Input: part model. Units: mm. Frame: model coordinates. A direction names the side the tool comes from. Round coordinates to 2 decimals unless told otherwise and drop trailing zeros. Order: outer loops, then holes, each group sorted by start corner. A loop starts at its lowest first (then second) coordinate and runs counter-clockwise, first axis right, second up. Notation, with made-up numbers: (53.5, 71) -> (68.5, 71) arc R21 cw to (68.5, 86) -> close; hole circle Ø7 at (-20, 23). An arc over 180 degrees is marked (long way). Use a Markdown table: item, result.
from build123d import *

# Parameters (mm, degrees)
SKETCH5_W             = 49.6
SKETCH5_H             = 24.3
SKETCH5_W_2           = 43.6
SKETCH5_H_2           = 18.3
BOSS_EXTRUDE3_DEPTH   = 7.5
FILLET1_R             = 3
SKETCH7_W             = 2.5
SKETCH7_H             = 2.5
BOSS_EXTRUDE5_DEPTH   = 4
SKETCH11_W            = 10
SKETCH11_H            = 4
BOSS_EXTRUDE6_DEPTH   = 12
FILLET3_R             = 3
SKETCH13_R            = 2.25
CUT_EXTRUDE1_DEPTH    = 56.377341937
CHAMFER2_SIZE         = 1
CHAMFER2_SIZE2        = 1.732050808
CIRPATTERN1_OUTLINE_R = 2.25
CIRPATTERN1_DEPTH     = 2.9999999
CIRPATTERN1_START     = 2.9999999
CIRPATTERN1_2_DEPTH   = 1.0000001
FILLET5_R             = 3
FILLET6_R             = 1


with BuildPart() as part:
    # Sketch5 → Boss-Extrude3 (new body)
    with BuildSketch(Plane(origin=(0, 0, 0), x_dir=(1, 0, 0), z_dir=(0, 1, 0))):
        with Locations((24.8, 12.15)):
            Rectangle(SKETCH5_W, SKETCH5_H)
        with Locations((24.8, 12.15)):
            Rectangle(SKETCH5_W_2, SKETCH5_H_2, mode=Mode.SUBTRACT)
    extrude(amount=BOSS_EXTRUDE3_DEPTH)

    # Fillet1
    fillet1_edges = [part.edges().sort_by_distance(p)[0] for p in [
        (49.6, 3.75, -24.3),
        (49.6, 3.75, 0),
        (0, 3.75, 0),
        (0, 3.75, -24.3),
    ]]
    fillet(fillet1_edges, radius=FILLET1_R)

    # Sketch7 → Boss-Extrude5 (add)
    with BuildSketch(Plane(origin=(0, 0, 0), x_dir=(1, 0, 0), z_dir=(0, 1, 0))):
        with Locations((45.35, 4.25)):
            Rectangle(SKETCH7_W, SKETCH7_H)
        with Locations((45.35, 20.05)):
            Rectangle(SKETCH7_W, SKETCH7_H)
        with Locations((4.25, 4.25)):
            Rectangle(SKETCH7_W, SKETCH7_H)
        with Locations((4.25, 20.05)):
            Rectangle(SKETCH7_W, SKETCH7_H)
    extrude(amount=BOSS_EXTRUDE5_DEPTH)

    # Sketch11 → Boss-Extrude6 (add)
    with BuildSketch(Plane.XY):
        with Locations((24.8, 2)):
            Rectangle(SKETCH11_W, SKETCH11_H)
    extrude(amount=BOSS_EXTRUDE6_DEPTH)

    # Fillet3
    fillet3_edges = [part.edges().sort_by_distance(p)[0] for p in [
        (19.8, 2, 0),
        (29.8, 2, 0),
        (24.8, 4, 0),
        (19.8, 2, 12),
        (29.8, 2, 12),
    ]]
    fillet(fillet3_edges, radius=FILLET3_R)

    # Sketch13 → Cut-Extrude1 (cut, through all)
    with BuildSketch(Plane(origin=(0, 4, 0), x_dir=(1, 0, 0), z_dir=(0, 1, 0))):
        with Locations(Location((24.8, -7, 0), (0, 0, 270))):
            Circle(SKETCH13_R)
    extrude(amount=-CUT_EXTRUDE1_DEPTH, mode=Mode.SUBTRACT)

    # Chamfer2
    chamfer2_edges = [part.edges().sort_by_distance(p)[0] for p in [
        (24.8, 4, 4.75),
    ]]
    chamfer2_side = [part.faces().sort_by_distance(p)[0] for p in [
        (24.8, 2, 4.75),
    ]]
    chamfer(chamfer2_edges, length=CHAMFER2_SIZE, length2=CHAMFER2_SIZE2, reference=chamfer2_side[0])

    # CirPattern1: read off the stored shape, not the designer's step
    # CirPattern1 outline → CirPattern1 (add)
    with BuildSketch(Plane(origin=(0, 0, 0), x_dir=(1, 0, 0), z_dir=(0, 1, 0))):
        with BuildLine():
            Line((19.8, 33.3), (19.8, 24.3))
            Line((19.8, 24.3), (29.8, 24.3))
            Line((29.8, 24.3), (29.8, 33.3))
            ThreePointArc((29.8, 33.3), (28.921320344, 35.421320344), (26.8, 36.3))
            Line((26.8, 36.3), (22.8, 36.3))
            ThreePointArc((22.8, 36.3), (20.678679656, 35.421320344), (19.8, 33.3))
        make_face()
        with Locations((24.8, 31.3)):
            Circle(CIRPATTERN1_OUTLINE_R, mode=Mode.SUBTRACT)
    extrude(amount=CIRPATTERN1_DEPTH)

    # CirPattern1 2 outline → CirPattern1 2 (add)
    with BuildSketch(Plane(origin=(0, 0, 0), x_dir=(1, 0, 0), z_dir=(0, 1, 0)).offset(CIRPATTERN1_START)):
        with BuildLine():
            Line((19.8, 33.3), (19.8, 24.3))
            Line((19.8, 24.3), (29.8, 24.3))
            Line((29.8, 24.3), (29.8, 33.3))
            ThreePointArc((29.8, 33.3), (28.921320344, 35.421320344), (26.8, 36.3))
            Line((26.8, 36.3), (22.8, 36.3))
            ThreePointArc((22.8, 36.3), (20.678679656, 35.421320344), (19.8, 33.3))
        make_face()
    extrude(amount=CIRPATTERN1_2_DEPTH)

    # CirPattern1 3 outline → CirPattern1 3 (revolve, cut)
    with BuildSketch(Plane(origin=(24.8, 0, -31.3), x_dir=(1, 0, 0), z_dir=(0, 0, 1))):
        Polygon((0, 2.9999999), (2.25, 2.9999999), (3.982050808, 4), (0, 4), align=None)
    revolve(axis=Axis((24.8, 0, -31.3), (0, 1, 0)), mode=Mode.SUBTRACT)

    # Fillet5
    fillet5_edges = [part.edges().sort_by_distance(p)[0] for p in [
        (29.8, 2, -24.3),
        (19.8, 2, -24.3),
        (24.8, 4, -24.3),
    ]]
    fillet(fillet5_edges, radius=FILLET5_R)

    # Fillet6
    fillet6_edges = [part.edges().sort_by_distance(p)[0] for p in [
        (5.5, 2, -18.8),
        (5.5, 2, -5.5),
        (44.1, 2, -5.5),
        (44.1, 2, -18.8),
    ]]
    fillet(fillet6_edges, radius=FILLET6_R)


solid = part.part
1) Pull-direction query (X, two-part tool) for faces 1 (the flat face through (46.6, 4, -12)), 2 (the cylindrical face through (31.11, 2.77, -24.82)), 3 (the flat face through (44.1, 2, -21)), 4 (the cylindrical face through (18.49, 2.77, 0.52)); classes: +X half, -X half, draft (parallel to the pull), parting line (faces both ways), or undercut.
Results found:
| item | result |
|---|---|
| face 1 | undercut |
| face 2 | +X half |
| face 3 | undercut |
| face 4 | -X half |
2) Cut plane B-B on z = 7. Return loops of the section in (x, y).
Results found:
| item | result |
|---|---|
| outline | (19.8, 0) -> (22.55, 0) -> (22.55, 3) -> (20.82, 4) -> (19.8, 4) -> close; (27.05, 0) -> (29.8, 0) -> (29.8, 4) -> (28.78, 4) -> (27.05, 3) -> close |
3) Set-up query: faces 5 (the flat face through (45, 4, -20)), 6 (the flat face through (19.8, 2, -30)), 7 (the flat face through (4, 2, -5.5)), 8 (the flat face through (19.8, 2, 6)). Return all of +Z, -Z, +X, -X, +Y, -Y with unobstructed straight access to the full face (end or side cutting, diameter ignored); none if empty.
Results found:
| item | result |
|---|---|
| face 5 | +Y |
| face 6 | -Z, -X, +Y, -Y |
| face 7 | +Y, -Y |
| face 8 | +Z, -X, +Y, -Y |
4) Pin query (flat end, axial travel): pin 1 Ø3 at (x, y) = (37, 6) entering from -Z; pin 2 Ø3 at (y, z) = (2, 5.5) entering from -X; pin 3 Ø2.5 at (x, z) = (24.8, 7) entering from +Y; pin 4 Ø4.5 at (x, z) = (27, -32.5) entering from +Y. Return the tip coordinate at first contact, or that it passes through.
Results found:
| item | result |
|---|---|
| pin 1 | stops at z = -24.3 |
| pin 2 | stops at x = 19.8 |
| pin 3 | passes through |
| pin 4 | stops at y = 4 |
5) Line query: L1, parallel to Z at x = 11.5, y = 3; L2, parallel to X at y = 0.75, z = 7; L3, parallel to Z at x = 32, y = 4. Output: solid intervals per line, ascending. Write a range as [from, to].
Results found:
| item | result |
|---|---|
| L1 | z = [-24.3, -21.3], [-3, 0] |
| L2 | x = [19.8, 22.55], [27.05, 29.8] |
| L3 | z = [-24.41, -21.3], [-3, 0.11] |
6) Cut plane C-C on x = 24.8. Count the separate pieces of the cut face and the enclosed holes in it, and give its area (3 significant figures).
Results found:
| item | result |
|---|---|
| separate pieces | 4 |
| enclosed holes | 0 |
| area | 105 mm² |
7) Cut plane A-A on x = 6.5. Return loops of the section in (y, z), and give its area (3 significant figures).
Results found:
| item | result |
|---|---|
| outline | (0, -24.3) -> (7.5, -24.3) -> (7.5, -21.3) -> (0, -21.3) -> close; (0, -3) -> (7.5, -3) -> (7.5, 0) -> (0, 0) -> close |
| area | 45.0 mm² |
